The listing builds one solid part. Answer for the finished solid, in the listing's coordinates (mm). Face numbers are marked on the shaded views. A direction names the side the tool comes from. Round coordinates to 2 decimals unless told otherwise and drop trailing zeros. Order: outer loops, then holes, each group sorted by start corner. A loop starts at its lowest first (then second) coordinate and runs counter-clockwise, first axis right, second up. Notation, with made-up numbers: (-29, -4) - (18, -4) arc R33 cw to (18, 28) - close; hole circle Ø3 at (31.25, -9). An arc over 180 degrees is marked (long way). One line per item, written item: value. Start each with the question number.
1. For a pull along Y with two mould halves and no side action, classify the marked faces 1, 2, 3 and 4 as released by +Y, released by -Y, zero draft, split by the parting line, or undercut.
2. Straight lines are drawn through the part: line 1 (Z direction, x = 3.5, y = 158); line 2 (X direction, y = 124.5, z = 7); line 3 (X direction, y = 28, z = 15.5). For each, find the intervals that lie inside material, in ascending order.
3. A tool of negligible diameter and unlimited length cuts with its end or side. For the marked faces 5 and 6, from which of +Z, -Z, +X, -X, +Y, -Y can it reach the whole face along a straight path? Write none if from no direction.
4. Flat-ended cylindrical pins translate along their axes: P1, Ø17.5, axis at x = 15, y = 156.5, coming from the +Z side; P2, Ø2, axis at y = 25.5, z = 10.5, coming from the +X side; P3, Ø8, axis at x = 7, y = 117, coming from the -Z side. Find the tip coordinate at first contact, or state that the pin passes through.
5. Section C-C, the plane y = 94.5 is taken. Give the vertices of the cut face in (x, z), then the cut area to 3 significant figures.
6. Section D-D, the plane z = 8.75 is taken. Give the vertices of the cut face in (x, y).
7. Section A-A, the plane x = -9 is taken. Give the vertices of the cut face in (y, z), then the cut area to 3 significant figures.
8. Section B-B, the plane z = 16 is taken. Give the vertices of the cut face in (x, y), then the cut area to 3 significant figures.
Autodesk Inventor part; units mm, degrees
ref_plane "YZ Plane" through (0, 0, 0) normal (1, 0, 0) x (0, 1, 0)
ref_plane "XZ Plane" through (0, 0, 0) normal (0, 1, 0) x (-1, 0, 0)
ref_plane "XY Plane" through (0, 0, 0) normal (0, 0, 1) x (1, 0, 0)
sketch "Эскиз1" plane through (0, 0, 0) normal (0, 0, 1) x (1, 0, 0)
  line L0 (-13, 0) -> (13, 0)
  line L1 (-47.5, 180) -> (47.5, 180)
  line L2 (-16.5, 130) -> (16.5, 130)
  line L3 (-12.9827, 110) -> (12.9827, 110)
  line L4 (-11.8003, 90) -> (11.8003, 90)
  line L5 (47.5, 180) -> (37.594, 168.7363)
  line L6 (-47.5, 180) -> (-37.594, 168.7363)
  line L7 (-37.594, 168.7363) -> (37.594, 168.7363)
  arc A0 (37.594, 168.7363) -> (12.9827, 110) centre (112.573, 102.7948) ccw
  arc A1 (12.9827, 110) -> (13, 0) centre (771.5375, 55.1194) ccw
  arc A2 (-12.9827, 110) -> (-37.594, 168.7363) centre (-112.573, 102.7948) ccw
  arc A3 (-13, 0) -> (-12.9827, 110) centre (-771.5375, 55.1194) ccw
  line L8 (-11, 80.4723) -> (-11, 26.1046)
  line L9 (11, 80.4723) -> (11, 26.1046)
  line L10 (-37.594, 168.7363) -> (13.0707, 111.1279)
  line L11 (37.594, 168.7363) -> (-13.0707, 111.1279)
  point P0 (0, 0)
  point P1 (0, 0)
  point P2 (0, 180)
  point P3 (0, 130)
  point P4 (0, 90)
  point P5 (0, 110)
  point P6 (-11, 55.1194)
  dimension "d0" = 26
  dimension "d1" = 95
  dimension "d2" = 33
  dimension "d5" = 180
  dimension "d6" = 50
  dimension "d7" = 20
  dimension "d8" = 20
  dimension "d9" = 15
  dimension "d10" = 15
  dimension "d13" = 22
  dimension "d19" = 55.1194
extrude "Выдавливание1" add sketch "Эскиз1" along normal blind 25
sketch "Эскиз2" plane through (0, 0, 0) normal (1, 0, 0) x (0, 1, 0)
  line L0 (0, 0) -> (110, 0)
  line L1 (110, 0) -> (110, 25)
  line L2 (0, 25) -> (110, 25)
  line L3 (0, 0) -> (0, 25)
  line L4 (110, 0) -> (169.3956, 0)
  line L5 (110, 25) -> (169.3956, 25)
  line L6 (110, 0) -> (110, 25)
  line L7 (130, 18) -> (130, 7)
  line L8 (55, 21) -> (55, 4)
  arc A0 (0, 25) -> (130, 18) centre (172.2556, 2013.3889) ccw
  arc A1 (130, 7) -> (0, 0) centre (172.2556, -1988.3889) ccw
  line L9 (180, 13) -> (180, 12)
  line L10 (145, 13) -> (145, 12)
  line L11 (180, 13) -> (145, 13)
  line L12 (180, 12) -> (145, 12)
  arc A2 (130, 18) -> (145, 13) centre (145, 38) ccw
  arc A3 (145, 12) -> (130, 7) centre (145, -13) ccw
  line L13 (168.7363, 0) -> (180, 0)
  line L14 (180, 0) -> (180, 25)
  line L15 (168.7363, 25) -> (180, 25)
  point P0 (130, 12.5)
  point P1 (0, 12.5)
  point P2 (55, 12.5)
  point P3 (180, 12.5)
  point P4 (169.3956, 12.5)
  point P5 (145, 12.5)
  point P6 (180, 12.5)
  dimension "d16" = 11
  dimension "d20" = 55
  dimension "d21" = 17
  dimension "d22" = 1
  dimension "d23" = 1
  dimension "d25" = 35
  dimension "d28" = 50
extrude "Выдавливание2" cut sketch "Эскиз2" along normal mid plane 100 contours L3 A0 L8 A1 | L8 A0 L1 A1 | L1 A0 L7 A1 | L7 A2 L10 A3 | L10 L11 L9 L12 keep common part
properties part number "bachi_v2"
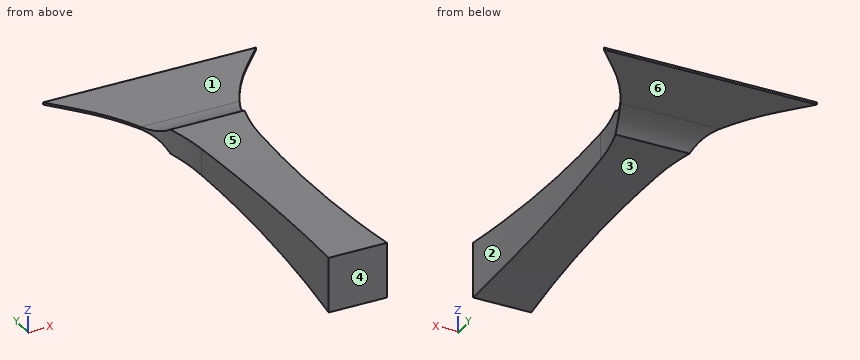
Answer list:
1. face 1: zero draft
1. face 2: undercut
1. face 3: released by +Y
1. face 4: released by -Y
2. line 1: z = 12 to 13
2. line 2: x = -15.11 to 15.11
2. line 3: x = -11.48 to 11.48
3. face 5: +Z, +X, -X, +Y
3. face 6: -Z, +X, -X, +Y
4. P1: stops at z = 13
4. P2: stops at x = 11.62
4. P3: stops at z = 6.57
5. outline: (-12.02, 5.93) - (12.02, 5.93) - (12.02, 19.07) - (-12.02, 19.07) - close
5. area: 316 mm²
6. outline: (-17.3, 132.67) arc R99.85 cw to (-12.98, 110) arc R760.53 cw to (-13, 0) - (13, 0) arc R760.54 cw to (12.98, 110) arc R99.85 cw to (17.3, 132.67) - close
7. outline: (0, 0) arc R1995.84 cw to (130, 7) arc R25 cw to (145, 12) - (180, 12) - (180, 13) - (145, 13) arc R25 cw to (130, 18) arc R1995.83 cw to (0, 25) - close
7. area: 2,250 mm²
8. outline: (-17.44, 133.13) arc R99.85 cw to (-12.98, 110) arc R760.53 cw to (-13, 0) - (13, 0) arc R760.54 cw to (12.98, 110) arc R99.85 cw to (17.44, 133.13) - close
8. area: 3,250 mm²
